Read the model definition and answer for the solid it produces. Units are mm, in the model's axes. A direction names the side the tool comes from. Give positions to 0.01 mm unless a question says otherwise; leave off trailing zeros. Write each loop counter-clockwise with the first axis right and the second up, starting at its lowest first coordinate (ties: lowest second). Pieces come first, ordered by that corner, then holes. Notation, with made-up numbers: M -10.5,-24.75 L 28.5,-24.75 A32 ccw 28.5,3.25 Z; hole C 43,77 d5. An arc over 180 degrees is marked long. Put each result on its own line as item: value.
from build123d import *

# Parameters (mm, degrees)
CUT_EXTRUDE1_DEPTH      = 9.926365442
CUT_EXTRUDE1_DEPTH_BACK = 9.926365442
SKETCH2_W               = 6.910571645
SKETCH2_H               = 0.8
SKETCH2_W_2             = 6.017195094
CHAMFER1_SIZE           = 0.4
CUT_EXTRUDE2_DEPTH      = 17.482718222
CUT_EXTRUDE2_DEPTH_BACK = 17.482718222
SKETCH3_R               = 1.2


with BuildPart() as part:
    # Sketch1 → Revolve1 (revolve)
    with BuildSketch(Plane.XY, mode=Mode.PRIVATE) as revolve1_sk:
        Polygon((-8, 0), (-8, 2.45), (-6.8, 2.45), (-6.8, 2.35), (-0.4, 2.35), (-0.4, 2.8), (0.4, 2.8), (0.4, 2.35), (6.8, 2.35), (6.8, 2.45), (8, 2.45), (8, 0), align=None)
    revolve(revolve1_sk.sketch.rotate(Axis((-8, 0, 0), (1, 0, 0)), 90), axis=Axis((-8, 0, 0), (1, 0, 0)))

    # Sketch2 → Cut-Extrude1 (cut, two sides: drawn at the far end of the back side and taken through both)
    with BuildSketch(Plane(origin=(0, 0, 0), x_dir=(1, 0, 0), z_dir=(0, 1, 0)).offset(-CUT_EXTRUDE1_DEPTH_BACK)):
        with Locations((-6.955285823, 0)):
            Rectangle(SKETCH2_W, SKETCH2_H)
        with Locations((6.508597547, 0)):
            Rectangle(SKETCH2_W_2, SKETCH2_H)
    extrude(amount=CUT_EXTRUDE1_DEPTH + CUT_EXTRUDE1_DEPTH_BACK, mode=Mode.SUBTRACT)

    # Chamfer1
    chamfer1_edges = [part.edges().sort_by_distance(p)[0] for p in [
        (8, 0, -2.45),
        (8, 0, 2.45),
        (-8, 0, -2.45),
        (-8, 0, 2.45),
    ]]
    chamfer(chamfer1_edges, length=CHAMFER1_SIZE)

    # Sketch3 → Cut-Extrude2 (cut, two sides: drawn at the far end of the back side and taken through both)
    with BuildSketch(Plane(origin=(8, 0, 0), x_dir=(0, 0, -1), z_dir=(1, 0, 0)).offset(-CUT_EXTRUDE2_DEPTH_BACK)):
        with Locations(Location((0, 0, 0), (0, 0, 289.471220634))):
            Circle(SKETCH3_R)
    extrude(amount=CUT_EXTRUDE2_DEPTH + CUT_EXTRUDE2_DEPTH_BACK, mode=Mode.SUBTRACT)


solid = part.part
(1) Section C-C on z = 0 is taken. Determine the outline of the cut face in (x, y), and give its area (3 significant figures).
Result:
outline: M -3.5,-2.35 L -0.4,-2.35 L -0.4,-2.8 L 0.4,-2.8 L 0.4,-2.35 L 3.5,-2.35 L 3.5,-1.2 L -3.5,-1.2 Z; M -3.5,1.2 L 3.5,1.2 L 3.5,2.35 L 0.4,2.35 L 0.4,2.8 L -0.4,2.8 L -0.4,2.35 L -3.5,2.35 Z
area: 16.8 mm²
(2) Given pin 1 Ø1 at (x, y) = (0.5, 1.5) entering from -Z; pin 2 Ø1 at (x, z) = (-1.5, -0.5) entering from +Y; pin 3 Ø1.4 at (x, y) = (7, -2) entering from -Z, each flat-ended and moving along its own axis, determine where each tip first touches the part or whether it passes through.
Result:
pin 1: stops at z = -2.61
pin 2: stops at y = 2.35
pin 3: stops at z = -2.08
(3) For a pull along Z with two mould halves and no side action, classify faces 5 (the face through (-7.19, 0.05, 2.45)), 6 (the face through (-6, 2, -0.4)), 7 (the face through (8, 0, 1.4)) as +Z half, -Z half, draft (parallel to the pull), parting line (faces both ways), or undercut.
Result:
face 5: +Z half
face 6: undercut
face 7: draft
(4) Section A-A on y = 0 is taken. Determine the outline of the cut face in (x, z), and give its area (3 significant figures).
Result:
outline: M -8,-2.05 L -7.6,-2.45 L -6.8,-2.45 L -6.8,-2.35 L -0.4,-2.35 L -0.4,-2.8 L 0.4,-2.8 L 0.4,-2.35 L 6.8,-2.35 L 6.8,-2.45 L 7.6,-2.45 L 8,-2.05 L 8,-1.2 L -8,-1.2 Z; M -8,1.2 L 8,1.2 L 8,2.05 L 7.6,2.45 L 6.8,2.45 L 6.8,2.35 L 0.4,2.35 L 0.4,2.8 L -0.4,2.8 L -0.4,2.35 L -6.8,2.35 L -6.8,2.45 L -7.6,2.45 L -8,2.05 Z
area: 37.7 mm²
(5) Which of the six approach directions +Z, -Z, +X, -X, +Y, -Y give full straight-line access (tool end or side, diameter ignored) to faces 1 (the face through (-3.5, 2, 0)), 2 (the face through (-7.19, -0.05, -2.45)), 3 (the face through (6, -2, -0.4)), 4 (the face through (7.21, 0.05, 2.45))?
Result:
face 1: -X, +Y, -Y
face 2: -Z, -X
face 3: +X, +Y, -Y
face 4: +Z, +X
(6) Section D-D on x = -0.25 is taken. Determine the outline of the cut face in (y, z).
Result:
outline: C 0,0 d5.6; hole C 0,0 d2.4
(7) Straight lines are drawn through the part: line 1 along Z through (x, y) = (-4.25, -0.2); line 2 along X through (y, z) = (1.1, 2.5); line 3 along Z through (x, y) = (3.5, 0.75). For each, find the intervals that lie inside material, in ascending order. Write a range as from..to.
Result:
line 1: z = -2.34..-1.18, 1.18..2.34
line 2: x = -0.4..0.4
line 3: z = -2.23..-0.94, 0.94..2.23
(8) Section B-B on x = -7 is taken. Determine the outline of the cut face in (y, z), and give its area (3 significant figures).
Result:
outline: M -2.42,-0.4 A2.45 ccw 2.42,-0.4 L 1.13,-0.4 A1.2 cw -1.13,-0.4 Z; M -2.42,0.4 L -1.13,0.4 A1.2 cw 1.13,0.4 L 2.42,0.4 A2.45 ccw Z
area: 12.3 mm²
